Autodesk Inventor part; units mm, degrees
ref_plane "YZ Plane" through (0, 0, 0) normal (1, 0, 0) x (0, 1, 0)
ref_plane "XZ Plane" through (0, 0, 0) normal (0, 1, 0) x (-1, 0, 0)
ref_plane "XY Plane" through (0, 0, 0) normal (0, 0, 1) x (1, 0, 0)
sketch "Sketch1" plane through (0, 0, 0) normal (0, 1, 0) x (-1, 0, 0)
  circle A0 centre (0, 0) radius 3
  dimension "d0" = 6
extrude "Extrusion1" add sketch "Sketch1" along normal blind 2.4
sketch "Sketch2" plane through (0, 2.4, 0) normal (0, 1, 0) x (1, 0, 0)
  line L0 (-1.55, 0.25) -> (1.55, 0.25)
  line L1 (1.55, 0.25) -> (1.55, -0.25)
  line L2 (1.55, -0.25) -> (-1.55, -0.25)
  line L3 (-1.55, -0.25) -> (-1.55, 0.25)
  line L4 (-0.25, -1.55) -> (0.25, -1.55)
  line L5 (0.25, -1.55) -> (0.25, 1.55)
  line L6 (0.25, 1.55) -> (-0.25, 1.55)
  line L7 (-0.25, 1.55) -> (-0.25, -1.55)
  point P0 (0, 0)
  dimension "d5" = 3.1
  dimension "d6" = 0.5
  dimension "d9" = 0.5
  dimension "d10" = 3.1
extrude "Extrusion2" cut sketch "Sketch2" against normal blind 1
fillet "Fillet1" radius 1 1 edges at (3, 2.4, 0)
sketch "Sketch3" plane through (0, 0, 0) normal (0, -1, 0) x (1, 0, 0)
  circle A0 centre (0, 0) radius 1.5
  dimension "d14" = 3
extrude "Extrusion3" add sketch "Sketch3" along normal blind 30
thread "Thread1"
properties part number "m3 30mm screw"
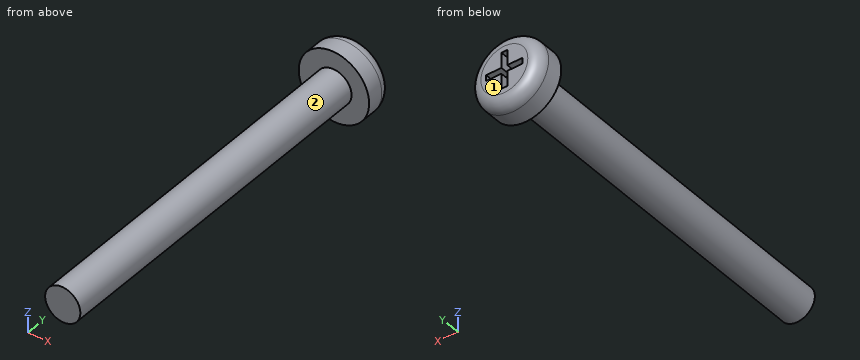
Check sheet for the modelled part. Datum: model origin and axes. Units: mm. Face numbers are marked on the shaded views. A direction names the side the tool comes from. Round coordinates to 2 decimals unless told otherwise and drop trailing zeros. Order: outer loops, then holes, each group sorted by start corner. A loop starts at its lowest first (then second) coordinate and runs counter-clockwise, first axis right, second up.
Q1. Set-up check for the marked faces 1 and 2: record each of +Z, -Z, +X, -X, +Y, -Y from which the full face is reachable in a straight line by a thin tool's end or side.
Filled sheet:
face 1: +Z, -Z, +X, -X, +Y
face 2: -Y
Q2. Depth check by flat-ended pin: P1, Ø1.1, axis at x = 0.5, y = 2, coming from the +Z side; P2, Ø0.6, axis at y = 2, z = 0, coming from the -X side; P3, Ø3, axis at y = -15.5, z = -1.5, coming from the -X side. Enter the tip coordinate at first touch or a pass-through.
Filled sheet:
P1: stops at z = 2.98
P2: stops at x = -2.95
P3: stops at x = -1.5
Q3. Scan lines: L1, parallel to Y at x = -0.55, z = 0; L2, parallel to Y at x = -1.65, z = 0; L3, parallel to Z at x = -0.05, y = -1. Record each from-to range of solid material in increasing order.
Filled sheet:
L1: y = -30 to 1.4
L2: y = 0 to 2.4
L3: z = -1.5 to 1.5
Q4. Cross-section at A-A, the plane y = -3. Enter the section's corners in (x, z).
Filled sheet:
outline: circle Ø3 at (0, 0)
